Here's how the part is built. I have some questions about the finished solid (model axes, mm). Face numbers are marked on the shaded views. A direction names the side the tool comes from. Give positions to 0.01 mm unless a question says otherwise; leave off trailing zeros. Loops run counter-clockwise (first coordinate to the right, second up) from the corner with the lowest first, then second, coordinate; pieces in that order, holes last.
Q1. Will these pins go through, and if not, where does the flat tip stop? P1, Ø1.1, axis at x = 10, z = 0.5, coming from the -Y side; P2, Ø0.5, axis at x = 14, z = 0.5, coming from the +Y side; P3, Ø6, axis at x = -5.5, y = -3, coming from the +Z side.
Q2. If we section it at C-C (z = 24.5): Please give me the cut outline in (x, y).
Q3. For the marked faces 1 and 2, which set-ups out of +Z, -Z, +X, -X, +Y, -Y let a thin tool reach every point of the face, with its end or its side?
Q4. I need wall thicknesses on line 1 (X direction, y = -1.5, z = 25); line 2 (Y direction, x = 18.8, z = 27); line 3 (Y direction, x = 0, z = 0.5). Which ranges of each line are inside material? Lowest first, please.
Q5. If we section it at B-B (x = 0): Please give me the cut outline in (y, z), plus the area to 3 significant figures.
Q6. We'd pull the mould along X, two halves only. Please class the marked faces 3, 4 and 5: +X half, -X half, draft (parallel to the pull), parting line (faces both ways), or undercut.
Q7. If we section it at A-A (y = 0): Please give me the cut outline in (x, z).
Q8. If we section it at D-D (y = 2.5): Please give me the cut outline in (x, z).
from build123d import *

# Parameters (mm, degrees)
SKETCH_1_R                = 3.25
EXTRUDE_1_DEPTH           = 1
HOLE_WIZARD_3_0_3_1_DEPTH = 1
SKETCH_7_R                = 1.25
EXTRUDE_2_DEPTH           = 1


# Read off the part's stored shape, not the designer's step: Ø3.0 (3) 直径槽口1
with BuildPart() as part:
    # 草图1 → 凸台-拉伸1 (new body)
    with BuildSketch(Plane.XY):
        with BuildLine():
            Line((11.56233108, 4.75), (19, 4.75))
            Line((19, 4.75), (19, -4.75))
            Line((19, -4.75), (11.56233108, -4.75))
            ThreePointArc((11.56233108, -4.75), (0, -12.5), (-11.56233108, -4.75))
            Line((-11.56233108, -4.75), (-19, -4.75))
            Line((-19, -4.75), (-19, 4.75))
            Line((-19, 4.75), (-11.56233108, 4.75))
            ThreePointArc((-11.56233108, 4.75), (0, 12.5), (11.56233108, 4.75))
        make_face()
        Circle(SKETCH_1_R, mode=Mode.SUBTRACT)
    extrude(amount=EXTRUDE_1_DEPTH)

    # Ø3.0 (3) 直径槽口1 outline → Ø3.0 (3) 直径槽口1 (cut)
    with BuildSketch(Plane.XY):
        with BuildLine():
            Line((7.5, -1.5), (12.5, -1.5))
            ThreePointArc((12.5, -1.5), (14, 0), (12.5, 1.5))
            Line((12.5, 1.5), (7.5, 1.5))
            ThreePointArc((7.5, 1.5), (6, 0), (7.5, -1.5))
        make_face()
        with BuildLine():
            ThreePointArc((-7.5, -1.5), (-6, 0), (-7.5, 1.5))
            Line((-7.5, 1.5), (-12.5, 1.5))
            ThreePointArc((-12.5, 1.5), (-14, 0), (-12.5, -1.5))
            Line((-12.5, -1.5), (-7.5, -1.5))
        make_face()
    extrude(amount=HOLE_WIZARD_3_0_3_1_DEPTH, mode=Mode.SUBTRACT)

    # 草图7 → 凸台-拉伸2 (add)
    with BuildSketch(Plane.ZY.offset(19)):
        with BuildLine():
            Line((1, 4.75), (27, 3.75))
            ThreePointArc((27, 3.75), (30.75, 0), (27, -3.75))
            Line((27, -3.75), (1, -4.75))
            Line((1, -4.75), (1, 4.75))
        make_face()
        with Locations((27, 0)):
            Circle(SKETCH_7_R, mode=Mode.SUBTRACT)
    extrude_2 = extrude(amount=-EXTRUDE_2_DEPTH)

    # 镜向1: 凸台-拉伸2 across plane
    add(extrude_2.mirror(Plane(origin=(0, 0, 0), x_dir=(0, 0, 1), z_dir=(1, 0, 0))))


solid = part.part
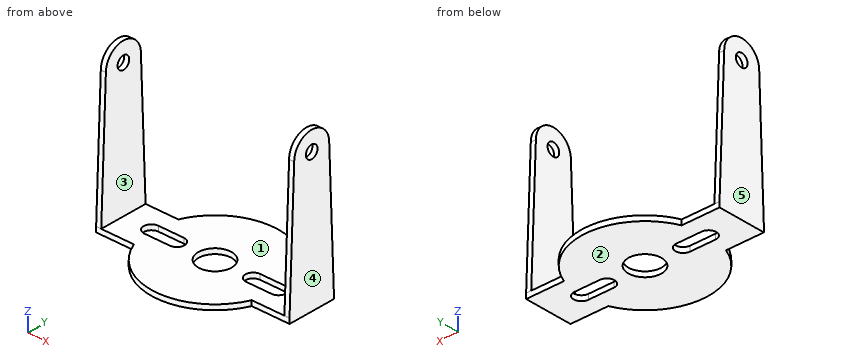
Check sheet entries:
1. P1: stops at y = -8.18
1. P2: stops at y = 4.75
1. P3: stops at z = 1
2. outline: (-19, -3.85) - (-18, -3.85) - (-18, 3.85) - (-19, 3.85) - close; (18, -3.85) - (19, -3.85) - (19, 3.85) - (18, 3.85) - close
3. face 1: +Z, +Y, -Y
3. face 2: -Z, +X, -X, +Y, -Y
4. line 1: x = -19 to -18, 18 to 19
4. line 2: y = -3.75 to -1.25, 1.25 to 3.75
4. line 3: y = -12.5 to -3.25, 3.25 to 12.5
5. outline: (-12.5, 0) - (-3.25, 0) - (-3.25, 1) - (-12.5, 1) - close; (3.25, 0) - (12.5, 0) - (12.5, 1) - (3.25, 1) - close
5. area: 18.5 mm2
6. face 3: undercut
6. face 4: +X half
6. face 5: -X half
7. outline: (-19, 0) - (-14, 0) - (-14, 1) - (-18, 1) - (-18, 25.75) - (-19, 25.75) - close; (-19, 28.25) - (-18, 28.25) - (-18, 30.75) - (-19, 30.75) - close; (-6, 0) - (-3.25, 0) - (-3.25, 1) - (-6, 1) - close; (3.25, 0) - (6, 0) - (6, 1) - (3.25, 1) - close; (14, 0) - (19, 0) - (19, 25.75) - (18, 25.75) - (18, 1) - (14, 1) - close; (18, 28.25) - (19, 28.25) - (19, 30.75) - (18, 30.75) - close
8. outline: (-19, 0) - (-2.08, 0) - (-2.08, 1) - (-18, 1) - (-18, 29.8) - (-19, 29.8) - close; (2.08, 0) - (19, 0) - (19, 29.8) - (18, 29.8) - (18, 1) - (2.08, 1) - close
